```python
from build123d import *

# Parameters (mm, degrees)
SKETCH1_R           = 2
BOSS_EXTRUDE1_DEPTH = 5
BOSS_EXTRUDE2_DEPTH = 35
CHAMFER1_SIZE       = 8
CHAMFER1_SIZE2      = 8.28424251


with BuildPart() as part:
    # Sketch1 → Boss-Extrude1 (new body)
    with BuildSketch(Plane.XY):
        Polygon((-14, 3.75), (14, 3.75), (14, -3.75), (-14, -3.75), (-59, -3.75), (-59, 3.75), align=None)
        with Locations((-10, 0)):
            Circle(SKETCH1_R, mode=Mode.SUBTRACT)
        with Locations((10, 0)):
            Circle(SKETCH1_R, mode=Mode.SUBTRACT)
    extrude(amount=BOSS_EXTRUDE1_DEPTH)

    # Sketch2 → Boss-Extrude2 (add)
    with BuildSketch(Plane.ZY.offset(59)):
        Polygon((0, 3.75), (0, 21.25), (-35, 21.25), (-35, 26.25), (5, 26.25), (5, 3.75), align=None)
    extrude(amount=-BOSS_EXTRUDE2_DEPTH)

    # Chamfer1
    chamfer1_edges = [part.edges().sort_by_distance(p)[0] for p in [
        (-24, 3.75, 2.5),
    ]]
    chamfer1_side = [part.faces().sort_by_distance(p)[0] for p in [
        (-24, 12.5, 0.458938994),
    ]]
    chamfer(chamfer1_edges, length=CHAMFER1_SIZE, length2=CHAMFER1_SIZE2, reference=chamfer1_side[0])


solid = part.part
```
The model under review builds one solid part; all positions refer to its coordinate system, in mm. A direction names the side the tool comes from. Coordinates: 2 decimals unless noted, no trailing zeros. Write each loop counter-clockwise with the first axis right and the second up, starting at its lowest first coordinate (ties: lowest second). Pieces come first, ordered by that corner, then holes. Notation, with made-up numbers: (67.5, 43.25) - (122.5, 43.25) arc R10 ccw to (122.5, 60.25) - close; hole circle Ø6 at (63, 8). An arc over 180 degrees is marked (long way). Answer in a Markdown table with one row per item. Add a question column.
Q1. To check wall thickness, follow line 1 along Y through (x, z) = (-10, 2.6); line 2 along Y through (x, z) = (-54, -9.5); line 3 along X through (y, z) = (20, 3). State the ranges of each line that lie inside material, in increasing order. Write a range as from..to.
Q2. For faces 1 (the face through (-24, 22, -10)), 2 (the face through (-42, 24, -35)), 3 (the face through (-42, 21.25, -17)), list the 3-axis set-ups (+Z, -Z, +X, -X, +Y, -Y) from which the entire face can be reached by the end or side of a thin tool; tool diameter is ignored.
Q3. Consider section C-C on x = -54. Give the boundary of the cut face in (y, z), then the cut area to 3 significant figures.
Q4. Clearance check with flat-ended pins moving along their axes: pin 1 (12 mm diameter, centred on y = 18.5, z = -16, fed in from +X); pin 2 (5 mm diameter, centred on x = -10, y = 0, fed in from -Z); pin 3 (3.5 mm diameter, centred on x = 10, y = 0, fed in from +Z); pin 4 (1.5 mm diameter, centred on x = -5.5, z = 1.5, fed in from +Y). State where each tip first meets the part, or that it passes through.
Q5. Draft analysis for pull direction Y (two halves, no side actions). For faces 4 (the face through (-31, 6, 0)), 5 (the face through (-23, -3.75, 2)), 6 (the face through (-11.6, -1.2, 2.5)), state which applies: +Y half, -Y half, draft (parallel to the pull), parting line (faces both ways), or undercut.
Q6. Consider section B-B on x = -10. Give the boundary of the cut face in (y, z), then the cut area to 3 significant figures.
Q7. Consider section A-A on y = 0. Give the boundary of the cut face in (x, z).
Q8. Consider section D-D on y = 24. Give the boundary of the cut face in (x, z).
Answers below:
| question | item | result |
|---|---|---|
| 1 | line 1 | -3.75..-2, 2..3.75 |
| 1 | line 2 | 21.25..26.25 |
| 1 | line 3 | -59..-24 |
| 2 | face 1 | +Z, -Z, +X, +Y |
| 2 | face 2 | -Z, +X, -X, +Y, -Y |
| 2 | face 3 | -Z, +X, -X, -Y |
| 3 | outline | (-3.75, 0) - (21.25, 0) - (21.25, -35) - (26.25, -35) - (26.25, 5) - (-3.75, 5) - close |
| 3 | area | 325 mm² |
| 4 | pin 1 | x = -24 |
| 4 | pin 2 | z = 0 |
| 4 | pin 3 | through |
| 4 | pin 4 | y = 3.75 |
| 5 | face 4 | draft |
| 5 | face 5 | -Y half |
| 5 | face 6 | undercut |
| 6 | outline | (-3.75, 0) - (-2, 0) - (-2, 5) - (-3.75, 5) - close; (2, 0) - (3.75, 0) - (3.75, 5) - (2, 5) - close |
| 6 | area | 17.5 mm² |
| 7 | outline | (-59, 0) - (-12, 0) - (-12, 5) - (-59, 5) - close; (-8, 0) - (8, 0) - (8, 5) - (-8, 5) - close; (12, 0) - (14, 0) - (14, 5) - (12, 5) - close |
| 8 | outline | (-59, -35) - (-24, -35) - (-24, 5) - (-59, 5) - close |
